The model under review builds one solid part; all positions refer to its coordinate system, in mm. Round coordinates to 2 decimals unless told otherwise and drop trailing zeros. Loops run counter-clockwise (first coordinate to the right, second up) from the corner with the lowest first, then second, coordinate; pieces in that order, holes last. Notation, with made-up numbers: (-5.75, 82.5) -> (44.25, 82.5) arc R28 ccw to (44.25, 102.5) -> close; hole circle Ø10 at (56, -11). An arc over 180 degrees is marked (long way). Use a Markdown table: item, result. Add a question column.
1) Wall thickness on probe 1 along X at (y, z) = (1041, -2); probe 2 along Z at (x, y) = (14.75, 862): over which ranges is each line inside the solid? List them lowest first.
2) Mouldability with a two-part tool opening along X and no side actions: class faces 1 (the flat face through (20, 580, -10)), 2 (the flat face through (0, 580, -10)), 3 (the flat face through (10, 1096, 0)) as released by +X, released by -X, zero draft, split by the parting line, or undercut.
3) Insertion check: pin 1 (2 mm diameter, centred on x = 12.5, z = -1.5, fed in from -Y); pin 2 (1.6 mm diameter, centred on x = 0.5, y = 1005.5, fed in from -Z); pin 3 (1.2 mm diameter, centred on x = 10, z = -2.5, fed in from +Y); pin 4 (0.8 mm diameter, centred on x = 19.5, y = 1006.5, fed in from +Z). Each pin has a flat end and moves straight along its axis. Give the tip position at first contact, or say it passes through.
4) Consider section B-B on y = 1026. Give the boundary of the cut face in (x, z), plus the area to 3 significant figures.
5) Consider section C-C on x = 15. Give the boundary of the cut face in (y, z), plus the area to 3 significant figures.
6) Consider section A-A on z = -11.75. Give the boundary of the cut face in (x, y), plus the area to 3 significant figures.
from build123d import *

# Parameters (mm, degrees)
SKETCH1_W           = 17
SKETCH1_H           = 17
BOSS_EXTRUDE1_DEPTH = 1177
SKETCH3_W           = 4
SKETCH3_H           = 20
CUT_EXTRUDE2_DEPTH  = 977
SKETCH2_W           = 4
SKETCH2_H           = 42.2
CUT_EXTRUDE1_DEPTH  = 1178.339798019


with BuildPart() as part:
    # Sketch1 → Boss-Extrude1 (new body)
    with BuildSketch(Plane(origin=(0, 0, 0), x_dir=(1, 0, 0), z_dir=(0, 1, 0))):
        with BuildLine():
            Line((0.5, 0), (19.5, 0))
            ThreePointArc((19.5, 0), (19.853553391, 0.146446609), (20, 0.5))
            Line((20, 0.5), (20, 19.5))
            ThreePointArc((20, 19.5), (19.853553391, 19.853553391), (19.5, 20))
            Line((19.5, 20), (0.5, 20))
            ThreePointArc((0.5, 20), (0.146446609, 19.853553391), (0, 19.5))
            Line((0, 19.5), (0, 0.5))
            ThreePointArc((0, 0.5), (0.146446609, 0.146446609), (0.5, 0))
        make_face()
        with Locations((10, 10)):
            Rectangle(SKETCH1_W, SKETCH1_H, mode=Mode.SUBTRACT)
    extrude(amount=BOSS_EXTRUDE1_DEPTH)

    # Sketch3 → Cut-Extrude2 (cut)
    with BuildSketch(Plane.ZY):
        with Locations((-2, 1167)):
            Rectangle(SKETCH3_W, SKETCH3_H)
        with Locations((-18, 1167)):
            Rectangle(SKETCH3_W, SKETCH3_H)
    cut_extrude2 = extrude(amount=-CUT_EXTRUDE2_DEPTH, mode=Mode.SUBTRACT)

    # Sketch2 → Cut-Extrude1 (cut, through all)
    with BuildSketch(Plane.ZY):
        with Locations((-2, 1015.9)):
            Rectangle(SKETCH2_W, SKETCH2_H)
        with Locations((-18, 1015.9)):
            Rectangle(SKETCH2_W, SKETCH2_H)
    cut_extrude1 = extrude(amount=-CUT_EXTRUDE1_DEPTH, mode=Mode.SUBTRACT)

    # Mirror1: Cut-Extrude2, Cut-Extrude1 across plane
    add(cut_extrude2.mirror(Plane.ZX.offset(588.5)), mode=Mode.SUBTRACT)
    add(cut_extrude1.mirror(Plane.ZX.offset(588.5)), mode=Mode.SUBTRACT)


solid = part.part
Result set:
| question | item | result |
|---|---|---|
| 1 | probe 1 | 0 to 1.5, 18.5 to 20 |
| 1 | probe 2 | -20 to -18.5, -1.5 to 0 |
| 2 | face 1 | released by +X |
| 2 | face 2 | released by -X |
| 2 | face 3 | zero draft |
| 3 | pin 1 | y = 20 |
| 3 | pin 2 | z = -16 |
| 3 | pin 3 | through |
| 3 | pin 4 | z = -4 |
| 4 | outline | (0, -16) -> (1.5, -16) -> (1.5, -4) -> (0, -4) -> close; (18.5, -16) -> (20, -16) -> (20, -4) -> (18.5, -4) -> close |
| 4 | area | 36.0 mm2 |
| 5 | outline | (20, -20) -> (140, -20) -> (140, -18.5) -> (20, -18.5) -> close; (20, -1.5) -> (140, -1.5) -> (140, 0) -> (20, 0) -> close; (182.2, -20) -> (994.8, -20) -> (994.8, -18.5) -> (182.2, -18.5) -> close; (182.2, -1.5) -> (994.8, -1.5) -> (994.8, 0) -> (182.2, 0) -> close; (1037, -20) -> (1157, -20) -> (1157, -18.5) -> (1037, -18.5) -> close; (1037, -1.5) -> (1157, -1.5) -> (1157, 0) -> (1037, 0) -> close |
| 5 | area | 3,160 mm2 |
| 6 | outline | (0, 0) -> (1.5, 0) -> (1.5, 1177) -> (0, 1177) -> close; (18.5, 0) -> (20, 0) -> (20, 1177) -> (18.5, 1177) -> close |
| 6 | area | 3,530 mm2 |
